Autodesk Fusion 360 part; units mm, degrees
sketch "Szkic1" plane through (0, 0, 0) normal (0, 0, 1) x (1, 0, 0)
  line L0 (-29, -30) -> (-29, 10)
  line L1 (31, -30) -> (-29, -30)
  line L2 (31, 10) -> (31, -30)
  line L3 (-29, 10) -> (31, 10)
  line L4 (10, -25) -> (10, -1.2)
  line L5 (10, -1.2) -> (-10, -1.2)
  line L6 (-10, -1.2) -> (-10, -25)
  line L7 (-10, -25) -> (10, -25)
  circle A0 centre (20, -20) radius 2
  circle A1 centre (20, 0) radius 2
  circle A2 centre (-15, 0) radius 2
  circle A3 centre (-15, -20) radius 2
  line L8 (-29, 10) -> (-29, -30)
  line L9 (-29, -30) -> (-35, -30)
  line L10 (-35, -30) -> (-35, 10)
  line L11 (-35, 10) -> (-29, 10)
  line L12 (31, 10) -> (31, -30)
  line L13 (31, -30) -> (45, -30)
  line L14 (45, -30) -> (45, 10)
  line L15 (45, 10) -> (31, 10)
  line L16 (45, -30) -> (45, -260)
  line L17 (-35, -30) -> (-35, -260)
  line L18 (-35, -260) -> (45, -260)
  circle A4 centre (-15, -20) radius 3.5
  circle A5 centre (-15, 0) radius 3.5
  circle A6 centre (20, 0) radius 3.5
  circle A7 centre (20, -20) radius 3.5
  dimension "d1" = 4
  dimension "d2" = 4
  dimension "d3" = 4
  dimension "d4" = 4
  dimension "d5" = 6
  dimension "d6" = 14
  dimension "d7" = 230
  dimension "d8" = 230
  dimension "d9" = 7
  dimension "d10" = 7
  dimension "d11" = 7
  dimension "d12" = 7
extrude "Wyciągnięcie proste1" add sketch "Szkic1" against normal blind 10 contours L0 L1 L2 L3 L8 L12 | L1 L9 L13 L16 L17 L18 | L2 L12 L13 L14 L15 | A4 | A5 | A6 | A7
extrude "Wyciągnięcie proste2" cut sketch "Szkic1" against normal blind 5 contours A4 | A5 | A6 | A7
sketch "Szkic2" plane through (0, 0, -10) normal (0, 0, -1) x (1, 0, 0)
  circle A0 centre (-15, 20) radius 2
  line L0 (-10, 25) -> (10, 25)
  line L1 (10, 25) -> (10, 1.2)
  line L2 (10, 1.2) -> (-10, 1.2)
  line L3 (-10, 1.2) -> (-10, 25)
  circle A1 centre (-15, 0) radius 2
  circle A2 centre (20, 0) radius 2
  circle A3 centre (20, 20) radius 2
  line L4 (-29, 30) -> (-29, -10)
  line L5 (-29, -10) -> (45, -10)
  line L6 (45, -10) -> (45, 260)
  line L7 (45, 260) -> (-35, 260)
  line L8 (-35, 260) -> (-35, 30)
  line L9 (-35, 30) -> (-29, 30)
  circle A4 centre (-25, 250) radius 1.75
  circle A5 centre (25, 250) radius 1.75
  circle A6 centre (-25, 200) radius 1.75
  circle A7 centre (-25, 150) radius 1.75
  circle A8 centre (-25, 100) radius 1.75
  circle A9 centre (-25, 50) radius 1.75
  circle A10 centre (-25, 250) radius 3.5
  circle A11 centre (25, 250) radius 3.5
  circle A12 centre (-25, 200) radius 3.5
  circle A13 centre (-25, 150) radius 3.5
  circle A14 centre (-25, 100) radius 3.5
  circle A15 centre (-25, 50) radius 3.5
  dimension "d17" = 3.5
  dimension "d18" = 3.5
  dimension "d19" = 3.5
  dimension "d20" = 3.5
  dimension "d21" = 3.5
  dimension "d22" = 3.5
  dimension "d23" = 7
  dimension "d24" = 7
  dimension "d25" = 7
  dimension "d26" = 7
  dimension "d27" = 7
  dimension "d28" = 7
extrude "Wyciągnięcie proste3" cut sketch "Szkic2" against normal blind 5 contours A10 | A11 | A12 | A13 | A14 | A15
extrude "Wyciągnięcie proste4" cut 6 faces at (-24.8702, -50.5687, -10) (-24.6044, -99.1189, -10) (-26.2448, -149.6385, -10) (-24.3128, -199.6032, -10) (-25.3003, -250.543, -10) (24.301, -249.4674, -10) along direction (0, 0, 1) blind 10
Check sheet for the modelled part. Datum: model origin and axes. Units: mm. A direction names the side the tool comes from. Give positions to 0.01 mm unless a question says otherwise; leave off trailing zeros. Answer as a JSON object with one key per item and string values. Group by question number.
1) Access from +Z, -Z, +X, -X, +Y, -Y to the whole of each face (thin tool, end or side, straight path). Record for faces 1 (the face through (4, -123, -10)), 2 (the face through (-25.759, -196.583, -7.535)), 3 (the face through (-13.12, -17.05, -2.46)), 4 (the face through (10, -13, -5)), 5 (the face through (7, 10, -5)).
2) Depth check by flat-ended pin: P1, Ø3.5, axis at x = -24, y = -100, coming from the -Z side; P2, Ø3.5, axis at x = -15.5, y = -21, coming from the +Z side; P3, Ø3, axis at x = -31.5, z = -7, coming from the +Y side. Enter the tip coordinate at first touch or a pass-through.
3) Sectioned sample at A-A (z = -7.25). Give the number of separate pieces and of enclosed holes in the cut face, then the cut area to 3 significant figures.
4) Thickness scan on probe 1 along Y at (x, z) = (-25, -2); probe 2 along Y at (x, z) = (-15, -3.25); probe 3 along Y at (x, z) = (-28, -6.75). Record the ranges inside material, lowest first. Write a range as from..to.
5) Release check for a two-part mould opening along X. For faces 6 (the face through (4, -123, 0)), 7 (the face through (23.34, 1.05, -2.46)) record: pulls with the +X half, pulls with the -X half, needs draft (parallel to the pull), parting line crosses it, or undercut.
Geometry results:
{
 "1": {"face 1": "-Z, +X, -X, +Y, -Y", "face 2": "-Z", "face 3": "+Z", "face 4": "+Z, -Z", "face 5": "+Z, -Z, +X, -X, +Y"},
 "2": {"P1": "stops at z = -5", "P2": "stops at z = -5", "P3": "stops at y = -30"},
 "3": {"separate pieces": "1", "enclosed holes": "11", "area": "20,600 mm^2"},
 "4": {"probe 1": "y = -260..-251.75, -248.25..-201.75, -198.25..-151.75, -148.25..-101.75, -98.25..-51.75, -48.25..10", "probe 2": "y = -260..-23.5, -16.5..-3.5, 3.5..10", "probe 3": "y = -260..-251.8, -248.2..-201.8, -198.2..-151.8, -148.2..-101.8, -98.2..-51.8, -48.2..10"},
 "5": {"face 6": "needs draft", "face 7": "undercut"}
}
